```python
from build123d import *

# Parameters (mm, degrees)
HOLE_WIZARD_6_5_6_5_1_D = 6.5


with BuildPart() as part:
    # 草圖1 → 旋轉1 (revolve)
    with BuildSketch(Plane.XY):
        Polygon((7, -8), (7, 8), (40, 8), (40, 5.5), (47.265, 5.5), (47.265, -5.5), (40, -5.5), (40, -8), align=None)
    revolve(axis=Axis((0, 49.340027701, 0), (0, -1, 0)))

    # 草圖7 → 旋轉2 (revolve)
    with BuildSketch(Plane.XY):
        Polygon((-49.5, -6.5), (-47.265, -5.5), (-40, -5.5), (-40, -6.5), (-47.265, -6.5), (-49.5, -7.5), align=None)
    revolve_2 = revolve(axis=Axis((0, 0, 0), (0, 1, 0)))

    # 鏡射1: 旋轉2 across plane
    add(revolve_2.mirror(Plane.ZX))

    # Ø6.5 (6.5) 直徑孔1 (through all)
    with Locations(Plane(origin=(0, 8, 0), x_dir=(1, 0, 0), z_dir=(0, 1, 0))):
        with Locations((-20.375, 20.375), (20.375, 20.375), (20.375, -20.375), (-20.375, -20.375), (0, 0)):
            Hole(HOLE_WIZARD_6_5_6_5_1_D / 2)


solid = part.part
```
For this review, take the finished solid that the model builds, in its own axes (mm). A direction names the side the tool comes from. Coordinates: 2 decimals unless noted, no trailing zeros. Loops run counter-clockwise (first coordinate to the right, second up) from the corner with the lowest first, then second, coordinate; pieces in that order, holes last. Notation, with made-up numbers: (-31.5, 71.25) -> (7.5, 71.25) arc R15 ccw to (7.5, 93.25) -> close; hole circle Ø7 at (-27.75, -13). An arc over 180 degrees is marked (long way). Return JSON: item names as keys, results as strings. Group by question number.
(1) Tool access review of faces 1 (the cylindrical face through (-8.67, 7.24, -39.05)), 2 (the flat face through (-39, -6.5, 11)), 3 (the cylindrical face through (45.08, -0.08, 14.2)), 4 (the cylindrical face through (23.62, -0.11, -20.52)), 5 (the flat face through (-8, 8, 1)): name each direction out of +Z, -Z, +X, -X, +Y, -Y from which nothing blocks a thin tool from reaching the whole face with its end or side.
(2) To check wall thickness, follow L1, parallel to Z at x = 0, y = 0.75 (3 decimals); L2, parallel to X at y = 3, z = -19; L3, parallel to Z at x = 18, y = -1.5. State the ranges of each line that lie inside material, in increasing order.
(3) Mouldability with a two-part tool opening along Z and no side actions: class faces 6 (the conical face through (-45.216, -6.563, 14.239)), 7 (the cylindrical face through (6.44, -6.99, 49.08)), 8 (the flat face through (8, -8, 1)) as pulls with the +Z half, pulls with the -Z half, needs draft (parallel to the pull), parting line crosses it, or undercut.
(4) Consider section B-B, the plane z = 0. Give the boundary of the cut face in (x, y) (3 decimals), plus the area to 3 significant figures.
(5) For pin 1 Ø5 at (x, y) = (19, 6) entering from -Z; pin 2 Ø1 at (x, y) = (3.5, -3) entering from +Z; pin 3 Ø8 at (x, y) = (-29.5, -5) entering from +Z, all flat-tipped, find the tip position at first contact; note any pin that passes through.
(6) Consider section A-A, the plane x = 0. Give the boundary of the cut face in (y, z) (3 decimals), plus the area to 3 significant figures.
(7) Consider section C-C, the plane y = -4. Give the boundary of the cut face in (x, z) (3 decimals), plus the area to 3 significant figures.
Results below:
{
 "1": {"face 1": "+Y", "face 2": "-Y", "face 3": "none", "face 4": "+Y, -Y", "face 5": "+Z, -Z, +X, -X, +Y"},
 "2": {"L1": "z = -47.265 to -7, 7 to 47.265", "L2": "x = -43.28 to -23.32, -17.43 to 17.43, 23.32 to 43.28", "L3": "z = -43.7 to -22.59, -18.16 to 18.16, 22.59 to 43.7"},
 "3": {"face 6": "undercut", "face 7": "parting line crosses it", "face 8": "needs draft"},
 "4": {"outline": "(-49.5, -7.5) -> (-47.265, -6.5) -> (-40, -6.5) -> (-40, -8) -> (-7, -8) -> (-7, 8) -> (-40, 8) -> (-40, 6.5) -> (-47.265, 6.5) -> (-49.5, 7.5) -> (-49.5, 6.5) -> (-47.265, 5.5) -> (-47.265, -5.5) -> (-49.5, -6.5) -> close; (7, -8) -> (40, -8) -> (40, -6.5) -> (47.265, -6.5) -> (49.5, -7.5) -> (49.5, -6.5) -> (47.265, -5.5) -> (47.265, 5.5) -> (49.5, 6.5) -> (49.5, 7.5) -> (47.265, 6.5) -> (40, 6.5) -> (40, 8) -> (7, 8) -> close", "area": "1,250 mm2"},
 "5": {"pin 1": "stops at z = -46.65", "pin 2": "stops at z = 47.17", "pin 3": "stops at z = 42.25"},
 "6": {"outline": "(-8, -40) -> (-6.5, -40) -> (-6.5, -47.265) -> (-7.5, -49.5) -> (-6.5, -49.5) -> (-5.5, -47.265) -> (5.5, -47.265) -> (6.5, -49.5) -> (7.5, -49.5) -> (6.5, -47.265) -> (6.5, -40) -> (8, -40) -> (8, -7) -> (-8, -7) -> close; (-8, 7) -> (8, 7) -> (8, 40) -> (6.5, 40) -> (6.5, 47.265) -> (7.5, 49.5) -> (6.5, 49.5) -> (5.5, 47.265) -> (-5.5, 47.265) -> (-6.5, 49.5) -> (-7.5, 49.5) -> (-6.5, 47.265) -> (-6.5, 40) -> (-8, 40) -> close", "area": "1,250 mm2"},
 "7": {"outline": "circle Ø94.53 at (0, 0); hole circle Ø6.5 at (-20.375, -20.375); hole circle Ø6.5 at (-20.375, 20.375); hole circle Ø14 at (0, 0); hole circle Ø6.5 at (20.375, -20.375); hole circle Ø6.5 at (20.375, 20.375)", "area": "6,730 mm2"}
}
